Job drawing, mm, ordinate dimensions from the low corner. One solid piece. A direction names the side the tool comes from. Round coordinates to 2 decimals unless told otherwise and drop trailing zeros. Write each loop counter-clockwise with the first axis right and the second up, starting at its lowest first coordinate (ties: lowest second). Pieces come first, ordered by that corner, then holes.
1) Saw through at D-D (x = 24.5). Write the cut outline in (y, z), plus the area to 3 significant figures.
2) Saw through at A-A (z = 13). Write the cut outline in (x, y).
3) Saw through at C-C (y = 22). Write the cut outline in (x, z), plus the area to 3 significant figures.
4) Which spindle directions (+Z, -Z, +X, -X, +Y, -Y) get a long thin tool onto all of the face, cutting with end or side? Do the marked faces 1 and 2. Say none if no direction does.
5) Saw through at B-B (x = 34). Write the cut outline in (y, z), plus the area to 3 significant figures.
6) Flat gauge pins, fed straight in: pin 1 (4.5 mm diameter, centred on x = 37.5, y = 12, fed in from +Z); pin 2 (5 mm diameter, centred on x = 39, z = 18, fed in from +Y); pin 3 (9 mm diameter, centred on y = 31, z = 20.5, fed in from +X). Where does each tip first touch, or does it go through?
7) Wall check: probe 1 along Y at (x, z) = (16, 27); probe 2 along Z at (x, y) = (16.5, 31.5); probe 3 along X at (y, z) = (27, 27.5). Give the ranges that are in metal, low to high.
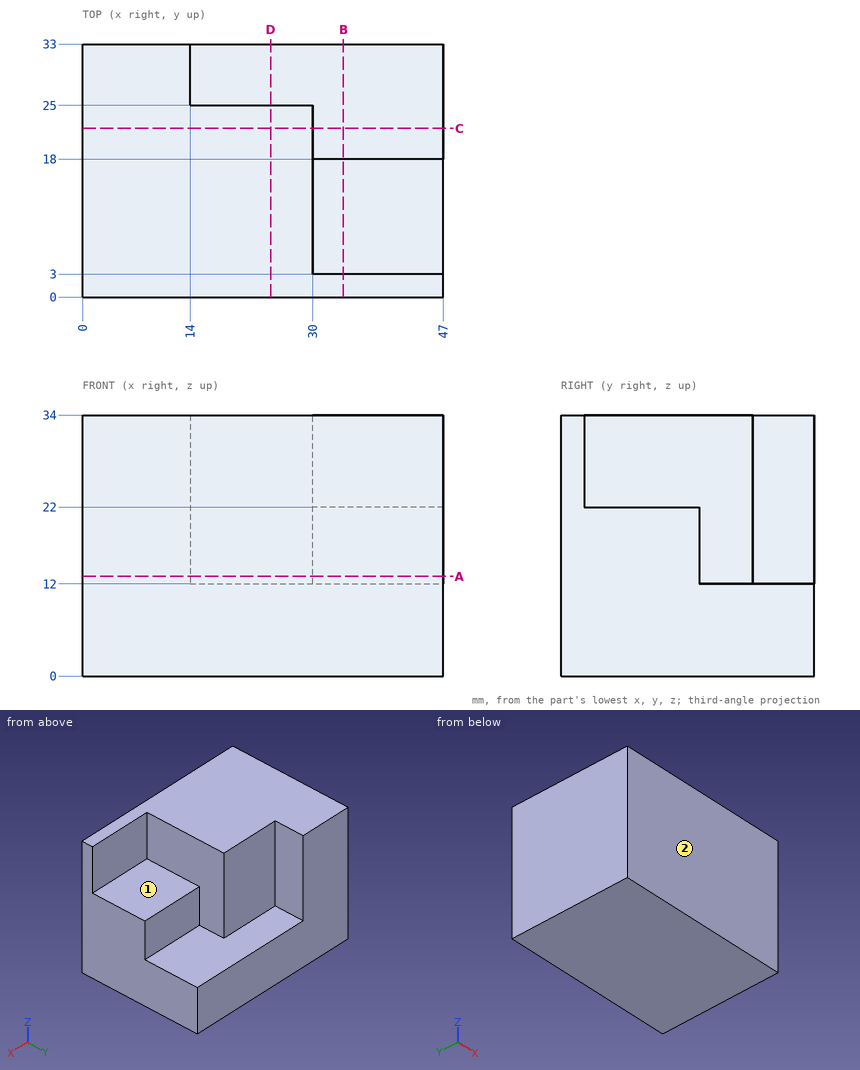
Evaluation:
1. outline: (0, 0) - (33, 0) - (33, 12) - (25, 12) - (25, 34) - (0, 34) - close
1. area: 946 mm2
2. outline: (0, 0) - (47, 0) - (47, 18) - (30, 18) - (30, 25) - (14, 25) - (14, 33) - (0, 33) - close
3. outline: (0, 0) - (47, 0) - (47, 12) - (30, 12) - (30, 34) - (0, 34) - close
3. area: 1,220 mm2
4. face 1: +Z, +X, +Y
4. face 2: +Z, -Z, +X, -X, -Y
5. outline: (0, 0) - (33, 0) - (33, 12) - (18, 12) - (18, 22) - (3, 22) - (3, 34) - (0, 34) - close
5. area: 612 mm2
6. pin 1: stops at z = 22
6. pin 2: stops at y = 18
6. pin 3: stops at x = 14
7. probe 1: y = 0 to 25
7. probe 2: z = 0 to 12
7. probe 3: x = 0 to 14
